For this review, take the finished solid that the model builds, in its own axes (mm). A direction names the side the tool comes from. Give positions to 0.01 mm unless a question says otherwise; leave off trailing zeros. Loops run counter-clockwise (first coordinate to the right, second up) from the corner with the lowest first, then second, coordinate; pieces in that order, holes last. Notation, with made-up numbers: (13, -3) - (39, -3) arc R30 cw to (39, 20) - close; hole circle Ø2 at (-4, 50). An arc over 180 degrees is marked (long way). Answer in a Markdown table with one row per item.
```python
from build123d import *
from build123d.topology import SkipClean

# Parameters (mm, degrees)
BOSS_EXTRUDE1_DEPTH  = 20
SKETCH2_W            = 53
SKETCH2_H            = 20
CUT_EXTRUDE1_DEPTH   = 20
FILLET1_R            = 9.75
FILLET1_OF_MIRROR4_R = 9.75
SKETCH4_R            = 2.1
CUT_EXTRUDE3_DEPTH   = 20


with BuildPart() as part:
    # Sketch1 → Boss-Extrude1 (new body)
    with BuildSketch(Plane(origin=(0, 0, 0), x_dir=(1, 0, 0), z_dir=(0, 1, 0))):
        with BuildLine():
            Line((34.641016151, 20), (90, 20))
            Line((90, 20), (90, -20))
            Line((90, -20), (34.641016151, -20))
            ThreePointArc((34.641016151, -20), (20, -34.641016151), (0, -40))
            Line((0, -40), (0, -20))
            Line((0, -20), (0, 20))
            Line((0, 20), (0, 40))
            ThreePointArc((0, 40), (20, 34.641016151), (34.641016151, 20))
        make_face()
    boss_extrude1 = extrude(amount=BOSS_EXTRUDE1_DEPTH)

    # Sketch2 → Cut-Extrude1 (cut)
    with BuildSketch(Plane(origin=(0, 20, 0), x_dir=(1, 0, 0), z_dir=(0, 1, 0))):
        with BuildLine():
            Line((0, 16), (0, -16))
            ThreePointArc((0, -16), (16, 0), (0, 16))
        make_face()
        with Locations((63.5, 0)):
            Rectangle(SKETCH2_W, SKETCH2_H)
    cut_extrude1 = extrude(amount=-CUT_EXTRUDE1_DEPTH, mode=Mode.SUBTRACT)

    # Fillet1
    fillet1_edges = [part.edges().sort_by_distance(p)[0] for p in [
        (90, 10, -20),
        (90, 10, 20),
    ]]
    fillet(fillet1_edges, radius=FILLET1_R)

    # Mirror4: Boss-Extrude1, Cut-Extrude1 across plane
    with SkipClean():  # the faces are left unmerged after this step: merging them gives an invalid solid
        add(boss_extrude1.mirror(Plane(origin=(0, 0, 0), x_dir=(0, 0, 1), z_dir=(1, 0, 0))))
        add(cut_extrude1.mirror(Plane(origin=(0, 0, 0), x_dir=(0, 0, 1), z_dir=(1, 0, 0))), mode=Mode.SUBTRACT)
    add(part.part.scale(1), mode=Mode.REPLACE)  # the faces are merged on a copy

    # Fillet1 of Mirror4
    fillet1_of_mirror4_edges = [part.edges().sort_by_distance(p)[0] for p in [
        (-90, 10, -20),
        (-90, 10, 20),
    ]]
    fillet(fillet1_of_mirror4_edges, radius=FILLET1_OF_MIRROR4_R)

    # Sketch4 → Cut-Extrude3 (cut)
    with BuildSketch(Plane(origin=(0, 20, 0), x_dir=(1, 0, 0), z_dir=(0, 1, 0))):
        with Locations(Location((21, 0, 0), (0, 0, 270))):
            Circle(SKETCH4_R)
        with Locations(Location((14.849242405, -14.849242405, 0), (0, 0, 270))):
            Circle(SKETCH4_R)
        with Locations(Location((0, -21, 0), (0, 0, 270))):
            Circle(SKETCH4_R)
        with Locations(Location((-14.849242405, -14.849242405, 0), (0, 0, 270))):
            Circle(SKETCH4_R)
        with Locations(Location((-21, 0, 0), (0, 0, 270))):
            Circle(SKETCH4_R)
        with Locations(Location((-14.849242405, 14.849242405, 0), (0, 0, 270))):
            Circle(SKETCH4_R)
        with Locations(Location((0, 21, 0), (0, 0, 270))):
            Circle(SKETCH4_R)
        with Locations(Location((14.849242405, 14.849242405, 0), (0, 0, 270))):
            Circle(SKETCH4_R)
    extrude(amount=-CUT_EXTRUDE3_DEPTH, mode=Mode.SUBTRACT)


solid = part.part
```
1. Clearance check with flat-ended pins moving along their axes: pin 1 (1.5 mm diameter, centred on y = 10, z = 14, fed in from -X); pin 2 (8 mm diameter, centred on y = 13.5, z = -5.5, fed in from -X); pin 3 (5 mm diameter, centred on x = -51, y = 10, fed in from -Z); pin 4 (6 mm diameter, centred on x = -45, z = 25.5, fed in from +Y). State where each tip first meets the part, or that it passes through.
Values:
| item | result |
|---|---|
| pin 1 | stops at x = -89.53 |
| pin 2 | stops at x = -37 |
| pin 3 | stops at z = -20 |
| pin 4 | passes through |
2. Wall thickness on line 1 (Z direction, x = 57, y = 18.75); line 2 (X direction, y = 15.75, z = -13); line 3 (X direction, y = 13.75, z = 0): over which ranges is each line inside the solid? List them lowest first. Write a range as [from, to].
Values:
| item | result |
|---|---|
| line 1 | z = [-20, -10], [10, 20] |
| line 2 | x = [-89.6, -15.84], [-13.85, -9.33], [9.33, 13.85], [15.84, 89.6] |
| line 3 | x = [-37, -23.1], [-18.9, -16], [16, 18.9], [23.1, 37] |
3. We need section B-B, the plane y = 17. Count the separate pieces of the cut face and the enclosed holes in it, and give its area (3 significant figures).
Values:
| item | result |
|---|---|
| separate pieces | 1 |
| enclosed holes | 9 |
| area | 6,050 mm^2 |
4. For faces 1 (the face through (58, 10, 20)), 2 (the face through (-37, 10, 0)), 3 (the face through (63, 10, 10)), list the 3-axis set-ups (+Z, -Z, +X, -X, +Y, -Y) from which the entire face can be reached by the end or side of a thin tool; tool diameter is ignored.
Values:
| item | result |
|---|---|
| face 1 | +Z, +X, +Y, -Y |
| face 2 | -X, +Y, -Y |
| face 3 | +X, +Y, -Y |
5. We need section D-D, the plane z = -28. Give the boundary of the cut face in (x, y).
Values:
| item | result |
|---|---|
| outline | (-28.57, 0) - (28.57, 0) - (28.57, 20) - (-28.57, 20) - close |
6. We need section A-A, the plane x = -58. Give the boundary of the cut face in (y, z).
Values:
| item | result |
|---|---|
| outline | (0, -20) - (20, -20) - (20, -10) - (0, -10) - close; (0, 10) - (20, 10) - (20, 20) - (0, 20) - close |
7. Mouldability with a two-part tool opening along Z and no side actions: class faces 4 (the face through (87.07, 10.14, 17.22)), 5 (the face through (-0.8, 10.14, 22.94)), 6 (the face through (-1, 20, 17)) as released by +Z, released by -Z, zero draft, split by the parting line, or undercut.
Values:
| item | result |
|---|---|
| face 4 | released by +Z |
| face 5 | undercut |
| face 6 | zero draft |
8. We need section C-C, the plane x = 21. Give the boundary of the cut face in (y, z).
Values:
| item | result |
|---|---|
| outline | (0, -34.04) - (20, -34.04) - (20, -2.1) - (0, -2.1) - close; (0, 2.1) - (20, 2.1) - (20, 34.04) - (0, 34.04) - close |
